Design review of the part built by this model. Coordinates are the model's own, in mm. Face numbers are marked on the shaded views. A direction names the side the tool comes from. Give positions to 0.01 mm unless a question says otherwise; leave off trailing zeros. Write each loop counter-clockwise with the first axis right and the second up, starting at its lowest first coordinate (ties: lowest second). Pieces come first, ordered by that corner, then holes. Notation, with made-up numbers: (-31, 62) -> (0, 62) arc R28 cw to (0, 83) -> close; hole circle Ø4 at (5.25, 21.5). An arc over 180 degrees is marked (long way). Return JSON: item names as keys, results as strings. Group by question number.
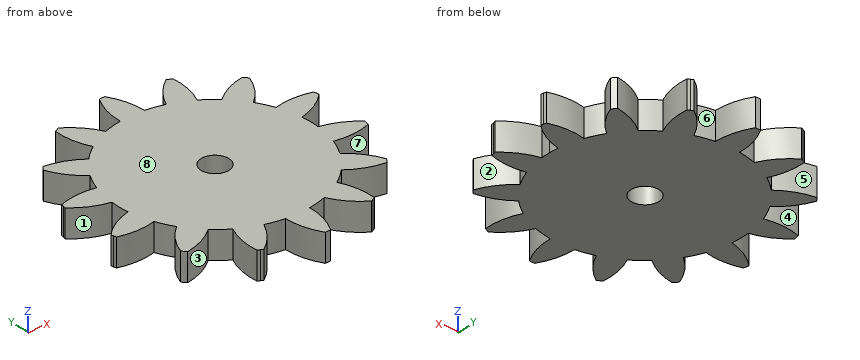
from build123d import *

# Parameters (mm, degrees)
F1_DEPTH = 2
F2_R     = 1
F3_DEPTH = 25


with BuildPart() as f1:
    # F0 (on Top) → F1 (new body)
    with BuildSketch(Plane.XY):
        with BuildLine():
            ThreePointArc((6.966901, -0.679915), (6.99172, -0.34036), (7, 0))
            ThreePointArc((7, 0), (6.99172, 0.34036), (6.966901, 0.679915))
            ThreePointArc((6.966901, 0.679915), (6.824495, 1.557647), (6.571965, 2.410243))
            ThreePointArc((6.571965, 2.410243), (6.306782, 3.037186), (5.981957, 3.635407))
            ThreePointArc((5.981957, 3.635407), (5.47282, 4.364429), (4.875371, 5.023023))
            ThreePointArc((4.875371, 5.023023), (4.364429, 5.47282), (3.812213, 5.870863))
            ThreePointArc((3.812213, 5.870863), (3.037186, 6.306782), (2.213149, 6.640931))
            ThreePointArc((2.213149, 6.640931), (1.557647, 6.824495), (0.887413, 6.943522))
            ThreePointArc((0.887413, 6.943522), (0, 7), (-0.887413, 6.943522))
            ThreePointArc((-0.887413, 6.943522), (-1.557647, 6.824495), (-2.213149, 6.640931))
            ThreePointArc((-2.213149, 6.640931), (-3.037186, 6.306782), (-3.812213, 5.870863))
            ThreePointArc((-3.812213, 5.870863), (-4.364429, 5.47282), (-4.875371, 5.023023))
            ThreePointArc((-4.875371, 5.023023), (-5.47282, 4.364429), (-5.981957, 3.635407))
            ThreePointArc((-5.981957, 3.635407), (-6.306782, 3.037186), (-6.571965, 2.410243))
            ThreePointArc((-6.571965, 2.410243), (-6.824495, 1.557647), (-6.966901, 0.679915))
            ThreePointArc((-6.966901, 0.679915), (-7, 0), (-6.966901, -0.679915))
            ThreePointArc((-6.966901, -0.679915), (-6.824495, -1.557647), (-6.571965, -2.410243))
            ThreePointArc((-6.571965, -2.410243), (-6.306782, -3.037186), (-5.981957, -3.635407))
            ThreePointArc((-5.981957, -3.635407), (-5.47282, -4.364429), (-4.875371, -5.023023))
            ThreePointArc((-4.875371, -5.023023), (-4.364429, -5.47282), (-3.812213, -5.870863))
            ThreePointArc((-3.812213, -5.870863), (-3.037186, -6.306782), (-2.213149, -6.640931))
            ThreePointArc((-2.213149, -6.640931), (-1.557647, -6.824495), (-0.887413, -6.943522))
            ThreePointArc((-0.887413, -6.943522), (0, -7), (0.887413, -6.943522))
            ThreePointArc((0.887413, -6.943522), (1.557647, -6.824495), (2.213149, -6.640931))
            ThreePointArc((2.213149, -6.640931), (3.037186, -6.306782), (3.812213, -5.870863))
            ThreePointArc((3.812213, -5.870863), (4.364429, -5.47282), (4.875371, -5.023023))
            ThreePointArc((4.875371, -5.023023), (5.47282, -4.364429), (5.981957, -3.635407))
            ThreePointArc((5.981957, -3.635407), (6.306782, -3.037186), (6.571965, -2.410243))
            ThreePointArc((6.571965, -2.410243), (6.824495, -1.557647), (6.966901, -0.679915))
        make_face()
        with BuildLine():
            ThreePointArc((6.571965, 2.410243), (6.824495, 1.557647), (6.966901, 0.679915))
            ThreePointArc((6.966901, 0.679915), (8.222094, 1.13804), (9.306319, 1.918963))
            Line((9.306319, 1.918963), (9.261815, 2.113949))
            Line((9.261815, 2.113949), (9.217311, 2.308934))
            ThreePointArc((9.217311, 2.308934), (7.901628, 2.542094), (6.571965, 2.410243))
        make_face()
        with BuildLine():
            ThreePointArc((9.306319, -1.918963), (8.222094, -1.13804), (6.966901, -0.679915))
            ThreePointArc((6.966901, -0.679915), (6.824495, -1.557647), (6.571965, -2.410243))
            ThreePointArc((6.571965, -2.410243), (7.901628, -2.542094), (9.217311, -2.308934))
            Line((9.217311, -2.308934), (9.261815, -2.113949))
            Line((9.261815, -2.113949), (9.306319, -1.918963))
        make_face()
        with BuildLine():
            ThreePointArc((4.875371, 5.023023), (5.47282, 4.364429), (5.981957, 3.635407))
            ThreePointArc((5.981957, 3.635407), (6.914074, 4.592771), (7.552097, 5.766787))
            Line((7.552097, 5.766787), (7.427399, 5.923153))
            Line((7.427399, 5.923153), (7.302701, 6.079519))
            ThreePointArc((7.302701, 6.079519), (6.016147, 5.718736), (4.875371, 5.023023))
        make_face()
        with BuildLine():
            ThreePointArc((7.552097, -5.766787), (6.914074, -4.592771), (5.981957, -3.635407))
            ThreePointArc((5.981957, -3.635407), (5.47282, -4.364429), (4.875371, -5.023023))
            ThreePointArc((4.875371, -5.023023), (6.016147, -5.718736), (7.302701, -6.079519))
            Line((7.302701, -6.079519), (7.427399, -5.923153))
            Line((7.427399, -5.923153), (7.552097, -5.766787))
        make_face()
        with BuildLine():
            ThreePointArc((2.213149, 6.640931), (3.037186, 6.306782), (3.812213, 5.870863))
            ThreePointArc((3.812213, 5.870863), (4.236636, 7.137848), (4.302089, 8.472427))
            Line((4.302089, 8.472427), (4.121896, 8.559204))
            Line((4.121896, 8.559204), (3.941702, 8.645981))
            ThreePointArc((3.941702, 8.645981), (2.939095, 7.762711), (2.213149, 6.640931))
        make_face()
        with BuildLine():
            ThreePointArc((4.302089, -8.472427), (4.236636, -7.137848), (3.812213, -5.870863))
            ThreePointArc((3.812213, -5.870863), (3.037186, -6.306782), (2.213149, -6.640931))
            ThreePointArc((2.213149, -6.640931), (2.939095, -7.762711), (3.941702, -8.645981))
            Line((3.941702, -8.645981), (4.121896, -8.559204))
            Line((4.121896, -8.559204), (4.302089, -8.472427))
        make_face()
        with BuildLine():
            ThreePointArc((-0.887413, 6.943522), (0, 7), (0.887413, 6.943522))
            ThreePointArc((0.887413, 6.943522), (0.720081, 8.269186), (0.2, 9.5))
            Line((0.2, 9.5), (0, 9.5))
            Line((0, 9.5), (-0.2, 9.5))
            ThreePointArc((-0.2, 9.5), (-0.720081, 8.269186), (-0.887413, 6.943522))
        make_face()
        with BuildLine():
            ThreePointArc((0.2, -9.5), (0.720081, -8.269186), (0.887413, -6.943522))
            ThreePointArc((0.887413, -6.943522), (0, -7), (-0.887413, -6.943522))
            ThreePointArc((-0.887413, -6.943522), (-0.720081, -8.269186), (-0.2, -9.5))
            Line((-0.2, -9.5), (0, -9.5))
            Line((0, -9.5), (0.2, -9.5))
        make_face()
        with BuildLine():
            ThreePointArc((-3.812213, 5.870863), (-3.037186, 6.306782), (-2.213149, 6.640931))
            ThreePointArc((-2.213149, 6.640931), (-2.939095, 7.762711), (-3.941702, 8.645981))
            Line((-3.941702, 8.645981), (-4.121896, 8.559204))
            Line((-4.121896, 8.559204), (-4.302089, 8.472427))
            ThreePointArc((-4.302089, 8.472427), (-4.236636, 7.137848), (-3.812213, 5.870863))
        make_face()
        with BuildLine():
            ThreePointArc((-3.941702, -8.645981), (-2.939095, -7.762711), (-2.213149, -6.640931))
            ThreePointArc((-2.213149, -6.640931), (-3.037186, -6.306782), (-3.812213, -5.870863))
            ThreePointArc((-3.812213, -5.870863), (-4.236636, -7.137848), (-4.302089, -8.472427))
            Line((-4.302089, -8.472427), (-4.121896, -8.559204))
            Line((-4.121896, -8.559204), (-3.941702, -8.645981))
        make_face()
        with BuildLine():
            ThreePointArc((-5.981957, 3.635407), (-5.47282, 4.364429), (-4.875371, 5.023023))
            ThreePointArc((-4.875371, 5.023023), (-6.016147, 5.718736), (-7.302701, 6.079519))
            Line((-7.302701, 6.079519), (-7.427399, 5.923153))
            Line((-7.427399, 5.923153), (-7.552097, 5.766787))
            ThreePointArc((-7.552097, 5.766787), (-6.914074, 4.592771), (-5.981957, 3.635407))
        make_face()
        with BuildLine():
            ThreePointArc((-7.302701, -6.079519), (-6.016147, -5.718736), (-4.875371, -5.023023))
            ThreePointArc((-4.875371, -5.023023), (-5.47282, -4.364429), (-5.981957, -3.635407))
            ThreePointArc((-5.981957, -3.635407), (-6.914074, -4.592771), (-7.552097, -5.766787))
            Line((-7.552097, -5.766787), (-7.427399, -5.923153))
            Line((-7.427399, -5.923153), (-7.302701, -6.079519))
        make_face()
        with BuildLine():
            ThreePointArc((-6.966901, 0.679915), (-6.824495, 1.557647), (-6.571965, 2.410243))
            ThreePointArc((-6.571965, 2.410243), (-7.901628, 2.542094), (-9.217311, 2.308934))
            Line((-9.217311, 2.308934), (-9.261815, 2.113949))
            Line((-9.261815, 2.113949), (-9.306319, 1.918963))
            ThreePointArc((-9.306319, 1.918963), (-8.222094, 1.13804), (-6.966901, 0.679915))
        make_face()
        with BuildLine():
            ThreePointArc((-9.217311, -2.308934), (-7.901628, -2.542094), (-6.571965, -2.410243))
            ThreePointArc((-6.571965, -2.410243), (-6.824495, -1.557647), (-6.966901, -0.679915))
            ThreePointArc((-6.966901, -0.679915), (-8.222094, -1.13804), (-9.306319, -1.918963))
            Line((-9.306319, -1.918963), (-9.261815, -2.113949))
            Line((-9.261815, -2.113949), (-9.217311, -2.308934))
        make_face()
    extrude(amount=F1_DEPTH)

    # F2 (on face) → F3 (cut)
    with BuildSketch(Plane.XY.offset(2)):
        Circle(F2_R)
    extrude(amount=-F3_DEPTH, mode=Mode.SUBTRACT)


solid = f1.part
Q1. Tool access review of the marked faces 1, 2, 3, 4 and 5: name each direction out of +Z, -Z, +X, -X, +Y, -Y from which nothing blocks a thin tool from reaching the whole face with its end or side.
Q2. Take a section at B-B, the plane x = 6.25. Give the boundary of the cut face in (y, z), plus the area to 3 significant figures.
Q3. Take a section at A-A, the plane y = -7.25. Give the boundary of the cut face in (x, z), plus the area to 3 significant figures.
Q4. Take a section at C-C, the plane x = 2.75. Give the boundary of the cut face in (y, z), plus the area to 3 significant figures.
Q5. For L1, parallel to Y at x = 0, z = 1; L2, parallel to X at y = -5.25, z = 0.5; L3, parallel to X at y = 8, z = 0.65, list the stretches that pass through material, from the lowest coordinate up. Write a range as from..to.
Q6. Take a section at D-D, the plane y = 1.5. Give the boundary of the cut face in (x, z).
Q7. Insertion check: pin 1 (1 mm diameter, centred on x = -3.5, z = 0.5, fed in from -Y); pin 2 (1 mm diameter, centred on x = 5, z = 0.5, fed in from +Y). Each pin has a flat end and moves straight along its axis. Give the tip position at first contact, or say it passes through.
Q8. Mouldability with a two-part tool opening along Y and no side actions: class the marked faces 6, 7 and 8 as +Y half, -Y half, draft (parallel to the pull), parting line (faces both ways), or undercut.
Final values:
{
 "1": {"face 1": "+Z, -Z, -X", "face 2": "+Z, -Z, +X", "face 3": "+Z, -Z, -Y", "face 4": "+Z, -Z", "face 5": "+Z, -Z, +Y"},
 "2": {"outline": "(-5.81, 0) -> (-3.86, 0) -> (-3.86, 2) -> (-5.81, 2) -> close; (-3.15, 0) -> (3.15, 0) -> (3.15, 2) -> (-3.15, 2) -> close; (3.86, 0) -> (5.81, 0) -> (5.81, 2) -> (3.86, 2) -> close", "area": "20.4 mm²"},
 "3": {"outline": "(-4.26, 0) -> (-2.55, 0) -> (-2.55, 2) -> (-4.26, 2) -> close; (-0.88, 0) -> (0.88, 0) -> (0.88, 2) -> (-0.88, 2) -> close; (2.55, 0) -> (4.26, 0) -> (4.26, 2) -> (2.55, 2) -> close", "area": "10.3 mm²"},
 "4": {"outline": "(-7.53, 0) -> (7.53, 0) -> (7.53, 2) -> (-7.53, 2) -> close", "area": "30.1 mm²"},
 "5": {"L1": "y = -9.5..-1, 1..9.5", "L2": "x = -7.32..-5.18, -4.63..4.63, 5.18..7.32", "L3": "x = -4.32..-3.16, -0.78..0.78, 3.16..4.32"},
 "6": {"outline": "(-8.8, 0) -> (8.8, 0) -> (8.8, 2) -> (-8.8, 2) -> close"},
 "7": {"pin 1": "stops at y = -8.65", "pin 2": "stops at y = 5.46"},
 "8": {"face 6": "+Y half", "face 7": "undercut", "face 8": "draft"}
}
